For this review, take the finished solid that the model builds, in its own axes (mm). A direction names the side the tool comes from. Round coordinates to 2 decimals unless told otherwise and drop trailing zeros. Write each loop counter-clockwise with the first axis right and the second up, starting at its lowest first coordinate (ties: lowest second). Pieces come first, ordered by that corner, then holes. Notation, with made-up numbers: (30.5, -14.5) - (34.5, -14.5) arc R14 ccw to (34.5, 7.5) - close; hole circle Ø11 at (65.5, 51). An arc over 180 degrees is marked (long way). One line per item, written item: value. Start each with the question number.
Q1. Add section C-C on x = 40.5. Write out the cut boundary in (y, z), and give its area (3 significant figures).
Q2. Add section D-D on y = -187.5. Give the number of separate pieces and of enclosed holes in the cut face, and give its area (3 significant figures).
Q3. Tool access review of faces 1 (the face through (-46.878, -196, 30)), 2 (the face through (2, -196, -11)), 3 (the face through (46.878, -196, 30)), 4 (the face through (46.878, -190, -14)), 5 (the face through (46.961, -190, 15)): name each direction out of +Z, -Z, +X, -X, +Y, -Y from which nothing blocks a thin tool from reaching the whole face with its end or side.
Q4. For probe 1 along X at (y, z) = (-190.25, 15); probe 2 along X at (y, z) = (-187.75, -14); probe 3 along Y at (x, z) = (20, -23), list the stretches that pass through material, from the lowest coordinate up.
Q5. Add section A-A on z = 9. Write out the cut boundary in (x, y), and give its area (3 significant figures).
Q6. Add section B-B on x = -20. Write out the cut boundary in (y, z), and give its area (3 significant figures).
Q7. Mouldability with a two-part tool opening along Z and no side actions: class faces 6 (the face through (-51, -190, 18.288)), 7 (the face through (51, -190, 10.974)), 8 (the face through (20.5, -196.3, 31.7)), 9 (the face through (51, -185.006, -15)) as +Z half, -Z half, draft (parallel to the pull), parting line (faces both ways), or undercut.
Q8. Clearance check with flat-ended pins moving along their axes: pin 1 Ø7 at (x, y) = (50.5, -189) entering from +Z; pin 2 Ø4.5 at (x, y) = (49.5, -192) entering from -Z; pin 3 Ø5.5 at (y, z) = (-187.5, -15) entering from -X. State where each tip first meets the part, or that it passes through.
```python
from build123d import *

# Parameters (mm, degrees)
SKETCH1_R           = 1.578396945
SKETCH1_W           = 79
SKETCH1_H           = 22
BOSS_EXTRUDE2_DEPTH = 2.54
BOSS_EXTRUDE3_DEPTH = 10


with BuildPart() as part:
    # Sketch1 → Boss-Extrude2 (new body)
    with BuildSketch(Plane(origin=(0, -197.546287398, 0), x_dir=(1, 0, 0), z_dir=(0, 1, 0))):
        with BuildLine():
            Line((-46.878416922, -25.602241557), (-46.878416922, -34.102241557))
            ThreePointArc((-46.878416922, -34.102241557), (-46.386819987, -35.289061544), (-45.2, -35.780658479))
            Line((-45.2, -35.780658479), (45.2, -35.780658479))
            ThreePointArc((45.2, -35.780658479), (46.386819987, -35.289061544), (46.878416922, -34.102241557))
            Line((46.878416922, -34.102241557), (46.878416922, -25.602241557))
            ThreePointArc((46.878416922, -25.602241557), (48.794516666, -20.66399163), (53.539905947, -18.310476992))
            add(Edge.make_bspline(
                [(53.539905947, -18.310476992), (53.808834541, -18.301511025), (54.349538715, -18.177417281), (55.023147103, -17.704797385), (55.473345475, -17.014152088), (55.578416916, -16.471377582), (55.578416922, -16.202870307)],
                knots=[0, 0, 0, 0, 0.001023741, 0.002047483, 0.003071224, 0.004094966, 0.004094966, 0.004094966, 0.004094966], degree=3))
            Line((55.578416922, -16.202870307), (55.578416922, 16.202870307))
            add(Edge.make_bspline(
                [(55.578416922, 16.202870307), (55.578416922, 16.417020125), (55.494048854, 16.850399632), (55.135979489, 17.398736831), (54.59856303, 17.775150348), (54.169613982, 17.873120493), (53.956037061, 17.880241063)],
                knots=[0, 0, 0, 0, 0.001023741, 0.002047483, 0.003071224, 0.004094966, 0.004094966, 0.004094966, 0.004094966], degree=3))
            ThreePointArc((53.956037061, 17.880241063), (48.93731184, 20.107602085), (46.878416939, 25.197758443))
            Line((46.878416939, 25.197758443), (46.878416939, 33.697758443))
            ThreePointArc((46.878416939, 33.697758443), (46.386819998, 34.884578436), (45.2, 35.376175365))
            Line((45.2, 35.376175365), (-45.2, 35.376175365))
            ThreePointArc((-45.2, 35.376175365), (-46.386819987, 34.88457843), (-46.878416922, 33.697758443))
            Line((-46.878416922, 33.697758443), (-46.878416922, 25.197758443))
            ThreePointArc((-46.878416922, 25.197758443), (-48.93731182, 20.107602071), (-53.956037052, 17.880241046))
            add(Edge.make_bspline(
                [(-53.956037052, 17.880241046), (-54.170067952, 17.873105344), (-54.600395569, 17.774343455), (-55.136497018, 17.398201742), (-55.494794219, 16.848541208), (-55.578416918, 16.416565886), (-55.578416922, 16.202870299)],
                knots=[0, 0, 0, 0, 0.001023741, 0.002047483, 0.003071224, 0.004094966, 0.004094966, 0.004094966, 0.004094966], degree=3))
            Line((-55.578416922, 16.202870299), (-55.578416922, -16.202870299))
            add(Edge.make_bspline(
                [(-55.578416922, -16.202870299), (-55.642358512, -16.407251091), (-55.69123907, -16.846051723), (-55.513228421, -17.476288615), (-55.112718518, -17.995994665), (-54.73258941, -18.21757272), (-54.530881465, -18.288139)],
                knots=[0, 0, 0, 0, 0.001023741, 0.002047483, 0.003071224, 0.004094966, 0.004094966, 0.004094966, 0.004094966], degree=3))
            ThreePointArc((-54.530881465, -18.288139), (-49.141195663, -20.309408908), (-46.878416922, -25.602241557))
        make_face()
        with Locations(Location((-20, 29.797758443, 0), (0, 0, 270))):
            Circle(SKETCH1_R, mode=Mode.SUBTRACT)
        with Locations(Location((-20, -30.202241557, 0), (0, 0, 270))):
            Circle(SKETCH1_R, mode=Mode.SUBTRACT)
        with Locations(Location((20, -30.202241557, 0), (0, 0, 270))):
            Circle(SKETCH1_R, mode=Mode.SUBTRACT)
        with Locations(Location((20.000000018, 29.79775846, 0), (0, 0, 270))):
            Circle(SKETCH1_R, mode=Mode.SUBTRACT)
        with Locations((2.5, 0)):
            Rectangle(SKETCH1_W, SKETCH1_H, mode=Mode.SUBTRACT)
    extrude(amount=BOSS_EXTRUDE2_DEPTH)

    # Sketch2 → Boss-Extrude3 (add)
    with BuildSketch(Plane(origin=(0, -195.006287398, 0), x_dir=(1, 0, 0), z_dir=(0, 1, 0))):
        with BuildLine():
            Line((-55.578416922, 16.202870299), (-55.578416922, -16.202870299))
            add(Edge.make_bspline(
                [(-55.578416922, -16.202870299), (-55.642358512, -16.407251091), (-55.69123907, -16.846051723), (-55.513228421, -17.476288615), (-55.112718518, -17.995994665), (-54.73258941, -18.21757272), (-54.530881465, -18.288139)],
                knots=[0, 0, 0, 0, 0.001023741, 0.002047483, 0.003071224, 0.004094966, 0.004094966, 0.004094966, 0.004094966], degree=3))
            Line((-54.530881465, -18.288139), (-46.878416922, -18.288139))
            Line((-46.878416922, -18.288139), (-46.878416922, 17.880241046))
            Line((-46.878416922, 17.880241046), (-53.956037052, 17.880241046))
            add(Edge.make_bspline(
                [(-53.956037052, 17.880241046), (-54.170067952, 17.873105344), (-54.600395569, 17.774343455), (-55.136497018, 17.398201742), (-55.494794219, 16.848541208), (-55.578416918, 16.416565886), (-55.578416922, 16.202870299)],
                knots=[0, 0, 0, 0, 0.001023741, 0.002047483, 0.003071224, 0.004094966, 0.004094966, 0.004094966, 0.004094966], degree=3))
        make_face()
        with BuildLine():
            Line((55.578416922, -10.974069665), (46.960695339, -10.974069665))
            Line((46.960695339, -10.974069665), (46.960695339, -18.310476992))
            Line((46.960695339, -18.310476992), (53.539905947, -18.310476992))
            add(Edge.make_bspline(
                [(53.539905947, -18.310476992), (53.808834541, -18.301511025), (54.349538715, -18.177417281), (55.023147103, -17.704797385), (55.473345475, -17.014152088), (55.578416916, -16.471377582), (55.578416922, -16.202870307)],
                knots=[0, 0, 0, 0, 0.001023741, 0.002047483, 0.003071224, 0.004094966, 0.004094966, 0.004094966, 0.004094966], degree=3))
            Line((55.578416922, -16.202870307), (55.578416922, -10.974069665))
        make_face()
        with BuildLine():
            Line((55.578416922, 10.999543279), (46.878416939, 10.999543279))
            Line((46.878416939, 10.999543279), (46.878416939, 18.098650861))
            Line((46.878416939, 18.098650861), (53.956037061, 17.880241063))
            add(Edge.make_bspline(
                [(55.578416922, 16.202870307), (55.578416922, 16.417020125), (55.494048854, 16.850399632), (55.135979489, 17.398736831), (54.59856303, 17.775150348), (54.169613982, 17.873120493), (53.956037061, 17.880241063)],
                knots=[0, 0, 0, 0, 0.001023741, 0.002047483, 0.003071224, 0.004094966, 0.004094966, 0.004094966, 0.004094966], degree=3))
            Line((55.578416922, 16.202870307), (55.578416922, 10.999543279))
        make_face()
    extrude(amount=BOSS_EXTRUDE3_DEPTH)


solid = part.part
```
Result set:
1. outline: (-197.55, -35.38) - (-195.01, -35.38) - (-195.01, -11) - (-197.55, -11) - close; (-197.55, 11) - (-195.01, 11) - (-195.01, 35.78) - (-197.55, 35.78) - close
1. area: 125 mm^2
2. separate pieces: 3
2. enclosed holes: 0
2. area: 436 mm^2
3. face 1: +Z, -X, +Y, -Y
3. face 2: +Y, -Y
3. face 3: +Z, +X, +Y, -Y
3. face 4: +Z, -Z, +Y
3. face 5: +Z, +Y
4. probe 1: x = -55.58 to -46.88, 46.96 to 55.58
4. probe 2: x = -55.58 to -46.88, 46.88 to 55.58
4. probe 3: y = -197.55 to -195.01
5. outline: (-55.58, -197.55) - (-37, -197.55) - (-37, -195.01) - (-46.88, -195.01) - (-46.88, -185.01) - (-55.58, -185.01) - close; (42, -197.55) - (55.58, -197.55) - (55.58, -195.01) - (42, -195.01) - close
5. area: 169 mm^2
6. outline: (-197.55, -35.38) - (-195.01, -35.38) - (-195.01, -31.38) - (-197.55, -31.38) - close; (-197.55, -28.22) - (-195.01, -28.22) - (-195.01, -11) - (-197.55, -11) - close; (-197.55, 11) - (-195.01, 11) - (-195.01, 28.62) - (-197.55, 28.62) - close; (-197.55, 31.78) - (-195.01, 31.78) - (-195.01, 35.78) - (-197.55, 35.78) - close
6. area: 109 mm^2
7. face 6: +Z half
7. face 7: undercut
7. face 8: undercut
7. face 9: draft
8. pin 1: stops at z = 18.31
8. pin 2: stops at z = -18.09
8. pin 3: stops at x = -55.58
